```python
from build123d import *

# Parameters (mm, degrees)
F0_R     = 1.4
F0_R_2   = 0.9
F0_R_3   = 3
F1_DEPTH = 5


with BuildPart() as f1:
    # F0 (on Front) → F1 (new body)
    with BuildSketch(Plane.XZ):
        with BuildLine():
            Line((-80, -6), (-11, -6))
            Line((-11, -6), (8, -6))
            Line((8, -6), (8, 6))
            Line((8, 6), (-11, 6))
            Line((-11, 6), (-80, 6))
            ThreePointArc((-80, 6), (-83.535534, 4.535534), (-85, 1))
            Line((-85, 1), (-85, -1))
            ThreePointArc((-85, -1), (-83.535534, -4.535534), (-80, -6))
        make_face()
        with Locations((-80, 0)):
            Circle(F0_R, mode=Mode.SUBTRACT)
        with Locations((-18, 0)):
            Circle(F0_R_2, mode=Mode.SUBTRACT)
        with Locations((-9, 0)):
            Circle(F0_R_2, mode=Mode.SUBTRACT)
        Circle(F0_R_3, mode=Mode.SUBTRACT)
    extrude(amount=F1_DEPTH)


solid = f1.part
```
For this review, take the finished solid that the model builds, in its own axes (mm). Round coordinates to 2 decimals unless told otherwise and drop trailing zeros. Write each loop counter-clockwise with the first axis right and the second up, starting at its lowest first coordinate (ties: lowest second). Pieces come first, ordered by that corner, then holes. Notation, with made-up numbers: (-28, -0.75) -> (30, -0.75) arc R23 ccw to (30, 27.25) -> close; hole circle Ø1 at (55, 68.5). An arc over 180 degrees is marked (long way). Use one line per item in the form item = value.
Q1. To check wall thickness, follow probe 1 along Z at (x, y) = (0, -2.35); probe 2 along Z at (x, y) = (-18, -3.1); probe 3 along X at (y, z) = (-2.85, -0.5). State the ranges of each line that lie inside material, in increasing order. Write a range as from..to.
Resolved:
probe_1 = -6..-3, 3..6
probe_2 = -6..-0.9, 0.9..6
probe_3 = -85..-81.31, -78.69..-18.75, -17.25..-9.75, -8.25..-2.96, 2.96..8
Q2. Consider section D-D (z = 4.75). State the section outline as (x, y) points.
Resolved:
outline = (-83.31, -5) -> (8, -5) -> (8, 0) -> (-83.31, 0) -> close
Q3. Consider section A-A (x = 0). State the section outline as (y, z) points, then the cut area to 3 significant figures.
Resolved:
outline = (-5, -6) -> (0, -6) -> (0, -3) -> (-5, -3) -> close; (-5, 3) -> (0, 3) -> (0, 6) -> (-5, 6) -> close
area = 30.0 mm²
Q4. Consider section B-B (z = 0). State the section outline as (x, y) points.
Resolved:
outline = (-85, -5) -> (-81.4, -5) -> (-81.4, 0) -> (-85, 0) -> close; (-78.6, -5) -> (-18.9, -5) -> (-18.9, 0) -> (-78.6, 0) -> close; (-17.1, -5) -> (-9.9, -5) -> (-9.9, 0) -> (-17.1, 0) -> close; (-8.1, -5) -> (-3, -5) -> (-3, 0) -> (-8.1, 0) -> close; (3, -5) -> (8, -5) -> (8, 0) -> (3, 0) -> close
Q5. Clearance check with a flat-ended pin moving along its axis: pin 1 Ø1.7 at (x, z) = (-80, 0) entering from -Y. State where the tip first meets the part, or that it passes through.
Resolved:
pin_1 = through
Q6. The part is to be moulded in two halves that separate along X. For faces 1 (the cylindrical face through (-8.14, -2.46, 0.27)), 2 (the flat face through (-39, 0, 0)), 3 (the flat face through (8, -2, 0)), 4 (the flat face through (-85, -2, 0)), say which applies: released by +X, released by -X, zero draft, split by the parting line, or undercut.
Resolved:
face_1 = undercut
face_2 = zero draft
face_3 = released by +X
face_4 = released by -X
Q7. Consider section C-C (y = -2). State the section outline as (x, z) points, then the cut area to 3 significant figures.
Resolved:
outline = (-85, -1) arc R5 ccw to (-80, -6) -> (8, -6) -> (8, 6) -> (-80, 6) arc R5 ccw to (-85, 1) -> close; hole circle Ø2.8 at (-80, 0); hole circle Ø1.8 at (-18, 0); hole circle Ø1.8 at (-9, 0); hole circle Ø6 at (0, 0)
area = 1,070 mm²
